```python
from build123d import *

# Parameters (mm, degrees)
F2_DEPTH = 25.4
F1_R     = 6.35
F3_DEPTH = 25.4
F4_DEPTH = 25.4


with BuildPart() as f2:
    # F0 (on Front) → F2 (new body)
    with BuildSketch(Plane.XZ):
        with BuildLine():
            ThreePointArc((-3.309767, 57.129443), (-19.570792, 48.808365), (-35.831816, 57.129443))
            ThreePointArc((-35.831816, 57.129443), (-51.061196, 53.756689), (-46.285682, 38.907315))
            ThreePointArc((-46.285682, 38.907315), (-32.008572, 26.752618), (-23.168363, 10.217104))
            ThreePointArc((-23.168363, 10.217104), (-11.073118, -3.064714), (0, 11.080521))
            ThreePointArc((0, 11.080521), (-0.335296, 29.39346), (9.641493, 44.753794))
            ThreePointArc((9.641493, 44.753794), (10.189797, 58.292246), (-3.309767, 57.129443))
        make_face()
    extrude(amount=F2_DEPTH)

    # F1 (on Front) → F3 (cut)
    with BuildSketch(Plane.XZ):
        with Locations((3.597573, 49.646493)):
            Circle(F1_R)
    extrude(amount=F3_DEPTH, mode=Mode.SUBTRACT)

    # F1 (on Front) → F4 (cut)
    with BuildSketch(Plane.XZ):
        with Locations((-41.875739, 48.49527)):
            Circle(F1_R)
    extrude(amount=-F4_DEPTH, mode=Mode.SUBTRACT)


solid = f2.part
```
Verification items for the finished model (mm, model axes). Coordinates: 2 decimals unless noted, no trailing zeros. Order: outer loops, then holes, each group sorted by start corner. A loop starts at its lowest first (then second) coordinate and runs counter-clockwise, first axis right, second up. Notation, with made-up numbers: (58, 51) - (75, 51) arc R27 cw to (75, 80) - close; hole circle Ø6 at (71.5, 8.5). An arc over 180 degrees is marked (long way). Return JSON: item names as keys, results as strings.
(1) Section check B-B, the plane y = -4.5. Record the cut outline in (x, z), and give its area (3 significant figures).
Filled sheet:
{"outline": "(-46.29, 38.91) arc R50.35 cw to (-23.17, 10.22) arc R11.76 ccw (long way) to (0, 11.08) arc R31.28 cw to (9.64, 44.75) arc R9.03 ccw (long way) to (-3.31, 57.13) arc R20.05 cw to (-35.83, 57.13) arc R10.55 ccw (long way) to start; hole circle Ø12.7 at (3.6, 49.65)", "area": "2,010 mm^2"}
(2) Thickness scan on line 1 along X through (y, z) = (-23, 48); line 2 along Z through (x, y) = (2, -8.75); line 3 along Z through (x, y) = (-15.5, -12). Record the ranges inside material, lowest first.
Filled sheet:
{"line 1": "x = -52.45 to -2.54, 9.73 to 12.16", "line 2": "z = 35.24 to 43.5, 55.79 to 60.58", "line 3": "z = -2.38 to 49.23"}
(3) Section check D-D, the plane x = -28. Record the cut outline in (y, z).
Filled sheet:
{"outline": "(-25.4, 21) - (0, 21) - (0, 50.67) - (-25.4, 50.67) - close"}
(4) Section check C-C, the plane z = 13. Record the cut outline in (x, y).
Filled sheet:
{"outline": "(-24.13, -25.4) - (-0.56, -25.4) - (-0.56, 0) - (-24.13, 0) - close"}
(5) Mould release check, pull along Z, two halves, no side actions. Record for faces 1 (the cylindrical face through (10.343, -12.522, 58.142)), 2 (the cylindrical face through (2.771, -12.522, 55.942)), 3 (the flat face through (-20, -25.4, 29)), 4 (the cylindrical face through (-0.406, -12.522, 29.143)): pulls with the +Z half, pulls with the -Z half, needs draft (parallel to the pull), parting line crosses it, or undercut.
Filled sheet:
{"face 1": "parting line crosses it", "face 2": "undercut", "face 3": "needs draft", "face 4": "undercut"}
(6) Section check A-A, the plane x = 6. Record the cut outline in (y, z), and give its area (3 significant figures).
Filled sheet:
{"outline": "(-25.4, 41.15) - (0, 41.15) - (0, 43.77) - (-25.4, 43.77) - close; (-25.4, 55.52) - (0, 55.52) - (0, 60.56) - (-25.4, 60.56) - close", "area": "194 mm^2"}
(7) Go/stop test with flat-tipped pins: pin 1 (2 mm diameter, centred on y = -15, z = 28, fed in from +X); pin 2 (1.5 mm diameter, centred on x = -7.5, y = -15, fed in from -Z); pin 3 (1.5 mm diameter, centred on x = -12.5, y = -7, fed in from +Z). Record where each tip stops, or that it passes through.
Filled sheet:
{"pin 1": "stops at x = -0.45", "pin 2": "stops at z = -2.61", "pin 3": "stops at z = 50.4"}
